Input: part model. Units: mm. Frame: model coordinates. A direction names the side the tool comes from. Coordinates: 2 decimals unless noted, no trailing zeros. Write each loop counter-clockwise with the first axis right and the second up, starting at its lowest first coordinate (ties: lowest second). Pieces come first, ordered by that corner, then holes. Notation, with made-up numbers: (-37, 11.25) - (-2, 11.25) arc R21 ccw to (-2, 50.25) - close; hole circle Ø8 at (74, 74). An arc over 180 degrees is marked (long way). Use a Markdown table: item, result. Add a question column.
Q1. Set-up query: faces 1 (the face through (30.051, -10.626, 13.858)), 2 (the face through (-7.871, -10.626, 13.858)), 3 (the face through (-12.7, -13, -1)). Return all of +Z, -Z, +X, -X, +Y, -Y with unobstructed straight access to the full face (end or side cutting, diameter ignored); none if empty.
Q2. Section query A-A (x = 33.5). Return the cut outline in (y, z) (1 decimal).
Q3. Material intervals for probe 1 along X at (y, z) = (53.5, -23); probe 2 along Z at (x, y) = (11.5, -7); probe 3 along Z at (x, y) = (2.5, -8.5), sorted ascending. Write a range as from..to.
Q4. Section query B-B (x = 12.5). Give the number of separate pieces and of enclosed holes in the cut face, then the cut area to 3 significant figures.
Q5. Pin query (flat end, axial travel): P1, Ø5, axis at x = 1, y = 29.5, coming from the +Z side; P2, Ø4, axis at x = 20.5, z = -35, coming from the +Y side; P3, Ø10, axis at x = 29.5, z = -23.5, coming from the +Y side; P4, Ø1.5, axis at x = 12.5, z = -36, coming from the +Y side. Return the tip coordinate at first contact, or that it passes through.
Q6. Mould query, pull axis Y, two halves, no side actions, for faces 4 (the face through (9.44, 45.98, 0.54)), 5 (the face through (9.39, 74.97, -32.19)), 6 (the face through (12.34, -12.4, 2.75)), 7 (the face through (0.905, 28.596, -35.342)). Classes: released by +Y, released by -Y, zero draft, split by the parting line, or undercut.
from build123d import *

# Parameters (mm, degrees)
SKETCH1_R           = 17.4625
SKETCH1_R_2         = 12.7
BOSS_EXTRUDE1_DEPTH = 12.7
SKETCH1_3_R         = 6.35
SKETCH1_3_R_2       = 12.7
BOSS_EXTRUDE2_DEPTH = 19.05
SKETCH1_4_R         = 17.4625
SKETCH1_4_R_2       = 12.7
BOSS_EXTRUDE3_DEPTH = 38.1
FILLET1_R           = 3.175


with BuildPart() as part:
    # Sketch1 → Boss-Extrude1 (new body)
    with BuildSketch(Plane(origin=(0, 0, 0), x_dir=(0, 0, -1), z_dir=(1, 0, 0))):
        Circle(SKETCH1_R)
        Circle(SKETCH1_R_2, mode=Mode.SUBTRACT)
    extrude(amount=-BOSS_EXTRUDE1_DEPTH)

    # Sketch1_3 → Boss-Extrude2 (add)
    with BuildSketch(Plane(origin=(0, 0, 0), x_dir=(0, 0, -1), z_dir=(1, 0, 0))):
        with BuildLine():
            Line((24.088040055, -8.057687403), (48.071506693, 63.6396466))
            ThreePointArc((48.071506693, 63.6396466), (39.894915337, 82.983138982), (19.681065043, 77.288615292))
            Line((19.681065043, 77.288615292), (-21.336666584, 13.780662505))
            ThreePointArc((-21.336666584, 13.780662505), (-11.005493886, -22.891900409), (24.088040055, -8.057687403))
        make_face()
        with Locations((33.016481658, 68.675701226)):
            Circle(SKETCH1_3_R, mode=Mode.SUBTRACT)
        Circle(SKETCH1_3_R_2, mode=Mode.SUBTRACT)
    extrude(amount=BOSS_EXTRUDE2_DEPTH)

    # Sketch1_4 → Boss-Extrude3 (add)
    with BuildSketch(Plane(origin=(0, 0, 0), x_dir=(0, 0, -1), z_dir=(1, 0, 0))):
        Circle(SKETCH1_4_R)
        Circle(SKETCH1_4_R_2, mode=Mode.SUBTRACT)
    extrude(amount=BOSS_EXTRUDE3_DEPTH)

    # Fillet1
    fillet1_edges = [part.edges().sort_by_distance(p)[0] for p in [
        (19.05, 45.534638899, 0.827800771),
        (0, -22.891900409, 11.005493886),
        (19.05, 82.983138982, -39.894915337),
        (19.05, -22.891900409, 11.005493886),
        (0, 27.790979598, -36.079773374),
        (0, 45.534638899, 0.827800771),
        (19.05, 0, 17.4625),
        (0, 0, 17.4625),
        (19.05, 27.790979598, -36.079773374),
        (0, 82.983138982, -39.894915337),
    ]]
    fillet(fillet1_edges, radius=FILLET1_R)


solid = part.part
Values follow:
| question | item | result |
|---|---|---|
| 1 | face 1 | +X |
| 1 | face 2 | -X |
| 1 | face 3 | +Z, -Z, -X, +Y, -Y |
| 2 | outline | circle Ø34.9 at (0, 0); hole circle Ø25.4 at (0, 0) |
| 3 | probe 1 | 0..19.05 |
| 3 | probe 2 | -24.44..-10.6, 10.6..24.42 |
| 3 | probe 3 | -23.86..-9.44, 9.44..23.86 |
| 4 | separate pieces | 1 |
| 4 | enclosed holes | 2 |
| 4 | area | 3,950 mm2 |
| 5 | P1 | z = 12.42 |
| 5 | P2 | y = 83.04 |
| 5 | P3 | through |
| 5 | P4 | y = 84.39 |
| 6 | face 4 | released by +Y |
| 6 | face 5 | undercut |
| 6 | face 6 | undercut |
| 6 | face 7 | released by -Y |
